Source: CAD feature listing. Evaluate the final solid. Frame: model axes, mm. A direction names the side the tool comes from. Give positions to 0.01 mm unless a question says otherwise; leave off trailing zeros. Loops run counter-clockwise (first coordinate to the right, second up) from the corner with the lowest first, then second, coordinate; pieces in that order, holes last. Notation, with made-up numbers: (-2.5, 75) -> (9.5, 75) arc R26 cw to (9.5, 109) -> close; hole circle Ø8 at (87.25, 18.5). An arc over 180 degrees is marked (long way). Return JSON: item names as keys, results as strings. Group by question number.
(1) Pin query (flat end, axial travel): pin 1 (3.5 mm diameter, centred on x = -0.5, y = 2, fed in from -Z); pin 2 (4 mm diameter, centred on y = 20, z = 6.5, fed in from -X); pin 3 (4 mm diameter, centred on x = 2, y = 15, fed in from +Z); pin 4 (8 mm diameter, centred on x = 9.5, y = 17.5, fed in from -Z). Return the tip coordinate at first contact, or that it passes through.
(2) Draft query along X for faces 6 (the face through (0.522, 12.035, 1.656)), 7 (the face through (11.923, 6.972, 3.755)), 8 (the face through (10, 5, -8)). Return one class per face: released by +X, released by -X, zero draft, split by the parting line, or undercut.
(3) Cut plane A-A on y = 18.5. Return loops of the section in (x, z).
(4) Cut plane B-B on y = 9.5. Return loops of the section in (x, z), then the cut area to 3 significant figures.
(5) Ray query, line 1 (Y direction, x = 1, z = 12.5); line 2 (X direction, y = 20.25, z = 0); line 3 (Y direction, x = -8, z = -13). Return the intervals inside material, ascending. Write a range as from..to.
(6) Access query for faces 1 (the face through (0, 1, 1)), 2 (the face through (-3.4, 9, -12.3)), 3 (the face through (-14.78, 2.46, 6.13)), 4 (the face through (9.76, 20.94, -2.17)), 5 (the face through (0, 0, -7)). Directions: +Z, -Z, +X, -X, +Y, -Y. A direction counts if a zero-diameter tool reaches every point of the face in a straight line with its end or side. Return the directions, or none.
Autodesk Inventor part; units mm, degrees
ref_plane "YZ Plane" through (0, 0, 0) normal (1, 0, 0) x (0, 1, 0)
ref_plane "XZ Plane" through (0, 0, 0) normal (0, 1, 0) x (-1, 0, 0)
ref_plane "XY Plane" through (0, 0, 0) normal (0, 0, 1) x (1, 0, 0)
sketch "草图1" plane through (0, 0, 0) normal (0, 1, 0) x (-1, 0, 0)
  circle A0 centre (0, 0) radius 16
  dimension "d0" = 32
extrude "拉伸1" add sketch "草图1" along normal blind 5
sketch "草图2" plane through (0, 0, 0) normal (0, -1, 0) x (1, 0, 0)
  line L0 (16, 1) -> (-16, 1)
  line L1 (-16, 1) -> (-16, -1)
  line L2 (-16, -1) -> (16, -1)
  line L3 (16, -1) -> (16, 1)
  line L4 (16, 1) -> (-16, -1) construction
  line L5 (-16, 1) -> (16, -1) construction
  point P0 (0, 0)
  dimension "d3" = 32
  dimension "d4" = 2
extrude "拉伸2" cut sketch "草图2" against normal blind 3
sketch "草图3" plane through (0, 5, 0) normal (0, 1, 0) x (1, 0, 0)
  circle A0 centre (0, 0) radius 12.5
  dimension "d7" = 25
extrude "拉伸3" add sketch "草图3" along normal blind 4
sketch "草图4" plane through (0, 9, 0) normal (0, 1, 0) x (1, 0, 0)
  circle A0 centre (0, 0) radius 15
  dimension "d10" = 30
extrude "拉伸4" add sketch "草图4" along normal blind 16
sketch "草图5" plane through (0, 25, 0) normal (0, 1, 0) x (1, 0, 0)
  circle A0 centre (0, 0) radius 10
  dimension "d13" = 20
hole "孔1" at (0, 25, 0) direction (0, -1, 0) diameter 20 depth 8 tip angle 118
sketch "草图6" plane through (0, 0, 0) normal (1, 0, 0) x (0, 1, 0)
  line L0 (9, 15) -> (25, 15)
  line L1 (24, 15) -> (25, 14)
  line L2 (25, -15) -> (25, 15)
  line L3 (-5, 0) -> (30, 0)
  point P0 (0, 0)
  dimension "d21" = 1
  dimension "d22" = 45
revolve "旋转1" cut sketch "草图6" angle 360 about axis through (0, -10, 0) along (0, 1, 0)
thread "螺纹1"
properties part number "2-螺塞" material "不锈钢"
Answers:
{
 "1": {"pin 1": "z = -16", "pin 2": "x = -14.31", "pin 3": "z = 15", "pin 4": "z = -13.96"},
 "2": {"face 6": "undercut", "face 7": "split by the parting line", "face 8": "zero draft"},
 "3": {"outline": "circle Ø30 at (0, 0); hole circle Ø20 at (0, 0)"},
 "4": {"outline": "circle Ø30 at (0, 0)", "area": "707 mm²"},
 "5": {"line 1": "0..5, 9..25", "line 2": "-15..-10, 10..15", "line 3": "0..5"},
 "6": {"face 1": "+X, -X, -Y", "face 2": "none", "face 3": "+Y, -Y", "face 4": "+Y", "face 5": "+Z, -Z, +X, -X, -Y"}
}
